Design review of the part shown in the three views and the two pictorial views. Dimensions are in mm from the part's minimum x, y and z. Round coordinates to 2 decimals unless told otherwise and drop trailing zeros. Write each loop counter-clockwise with the first axis right and the second up, starting at its lowest first coordinate (ties: lowest second). Pieces come first, ordered by that corner, then holes. Notation, with made-up numbers: (-0.75, -23) -> (56.25, -23) arc R18 ccw to (56.25, -8) -> close; hole circle Ø1 at (-1, 68.5). An arc over 180 degrees is marked (long way). One line per question, with ' | ' between items. Start each with the question number.
1) Consider section A-A (x = 12.5). Give the boundary of the cut face in (y, z), then the cut area to 3 significant figures.
2) Insertion check: pin 1 Ø8 at (x, z) = (12.5, 147.5) entering from +Y; pin 2 Ø4.5 at (x, z) = (12.5, 80) entering from +Y. Each pin has a flat end and moves straight along its axis. Give the tip position at first contact, or say it passes through.
3) Consider section B-B (z = 80). Give the boundary of the cut face in (x, y), then the cut area to 3 significant figures.
4) For probe 1 along Z at (x, y) = (12.5, 4); probe 2 along X at (y, z) = (2.6, 147.5); probe 3 along Z at (x, y) = (14.25, 0.6), list the stretches that pass through material, from the lowest coordinate up.
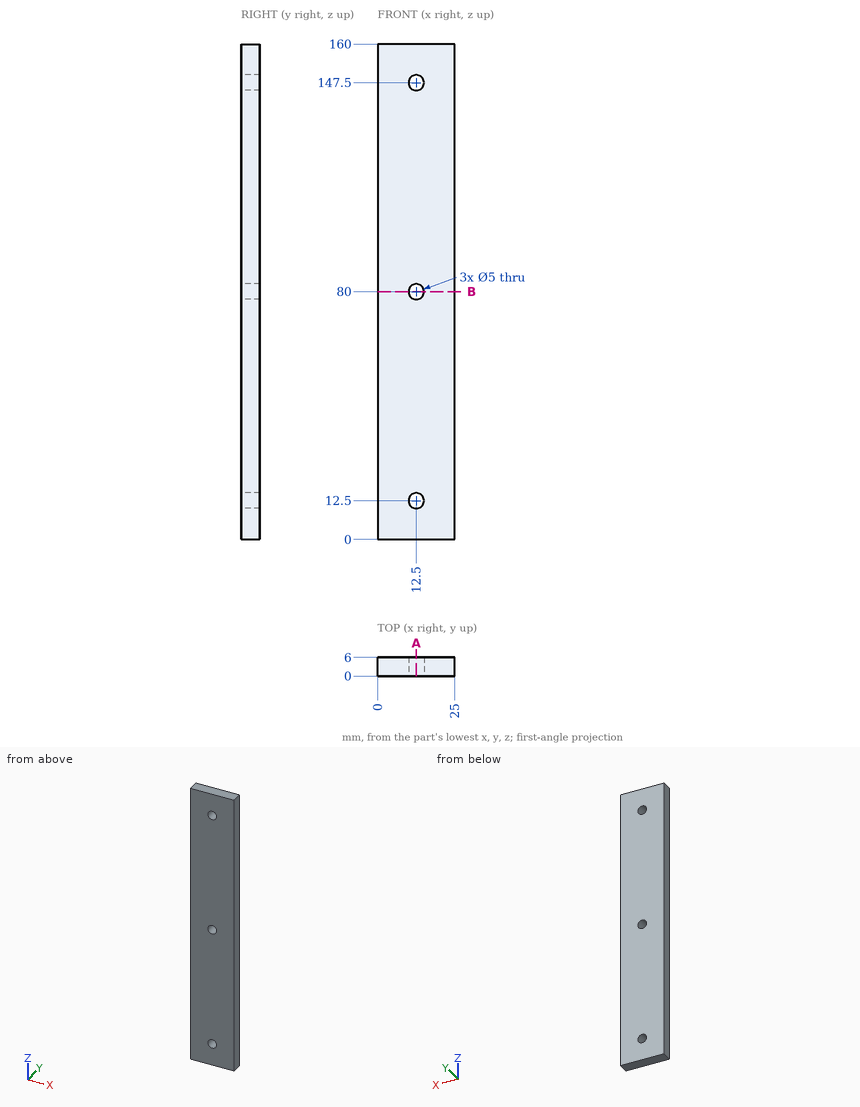
From the geometry:
1) outline: (0, 0) -> (6, 0) -> (6, 10) -> (0, 10) -> close; (0, 15) -> (6, 15) -> (6, 77.5) -> (0, 77.5) -> close; (0, 82.5) -> (6, 82.5) -> (6, 145) -> (0, 145) -> close; (0, 150) -> (6, 150) -> (6, 160) -> (0, 160) -> close | area: 870 mm2
2) pin 1: stops at y = 6 | pin 2: passes through
3) outline: (0, 0) -> (10, 0) -> (10, 6) -> (0, 6) -> close; (15, 0) -> (25, 0) -> (25, 6) -> (15, 6) -> close | area: 120 mm2
4) probe 1: z = 0 to 10, 15 to 77.5, 82.5 to 145, 150 to 160 | probe 2: x = 0 to 10, 15 to 25 | probe 3: z = 0 to 10.71, 14.29 to 78.21, 81.79 to 145.71, 149.29 to 160
